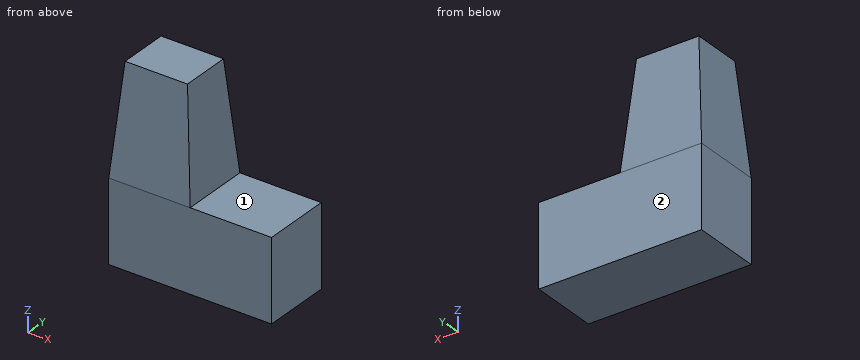
```python
from build123d import *

# Parameters (mm, degrees)
F0_W     = 60
F0_H     = 30
F1_DEPTH = 25.4
F2_W     = 30
F2_H     = 25.4
F3_DEPTH = 40
F3_TAPER = 5


with BuildPart() as f1:
    # F0 (on Front) → F1 (new body)
    with BuildSketch(Plane.XZ):
        with Locations((-10.6705549789, -15)):
            Rectangle(F0_W, F0_H)
    extrude(amount=F1_DEPTH)

    # F2 (on face) → F3 (join)
    with BuildSketch(Plane.XY):
        with Locations((-25.6705549789, -12.7)):
            Rectangle(F2_W, F2_H)
    extrude(amount=F3_DEPTH, taper=F3_TAPER)


solid = f1.part
```
Source: CAD feature listing. Evaluate the final solid. Frame: model axes, mm. Face numbers are marked on the shaded views. A direction names the side the tool comes from. Coordinates: 2 decimals unless noted, no trailing zeros. Loops run counter-clockwise (first coordinate to the right, second up) from the corner with the lowest first, then second, coordinate; pieces in that order, holes last. Notation, with made-up numbers: M -21.5,-32.75 L -10.5,-32.75 A24 ccw -10.5,-19.75 Z; hole C 68,-37 d11. An arc over 180 degrees is marked long. Put each result on its own line as item: value. Start each with the question number.
1) Cut plane D-D on x = 11. Return the cut outline in (y, z), then the cut area to 3 significant figures.
2) Reachability of the marked faces 1 and 2 from +Z, -Z, +X, -X, +Y, -Y: full face, straight path, thin tool, end or side. Return the list, or none.
3) Cut plane B-B on x = -26. Return the cut outline in (y, z).
4) Cut plane C-C on z = 14.5. Return the cut outline in (x, y), then the cut area to 3 significant figures.
5) Cut plane A-A on y = -16.75. Return the cut outline in (x, z).
6) Ray query, L1, parallel to Z at x = 8, y = -13.25; L2, parallel to X at y = -14.5, z = 12; L3, parallel to X at y = -13, z = 10.5. Return the intervals inside material, ascending. Write a range as from..to.
7) Contact query for flat-ended pins moving along their axis: pin 1 Ø4 at (y, z) = (-3, 11.5) entering from -X; pin 2 Ø3 at (x, y) = (-2.5, -16.5) entering from +Z; pin 3 Ø1 at (y, z) = (-18, 22.5) entering from -X. Output: stop coordinate, or through.
The answers:
1. outline: M -25.4,-30 L 0,-30 L 0,0 L -25.4,0 Z
1. area: 762 mm²
2. face 1: +Z, +X, +Y, -Y
2. face 2: +Z, -Z, +X, -X, +Y
3. outline: M -25.4,-30 L 0,-30 L 0,0 L -3.5,40 L -21.9,40 L -25.4,0 Z
4. outline: M -39.4,-24.13 L -11.94,-24.13 L -11.94,-1.27 L -39.4,-1.27 Z
4. area: 628 mm²
5. outline: M -40.67,-30 L 19.33,-30 L 19.33,0 L -10.67,0 L -14.17,40 L -37.17,40 L -40.67,0 Z
6. L1: z = -30..0
6. L2: x = -39.62..-11.72
6. L3: x = -39.75..-11.59
7. pin 1: stops at x = -39.84
7. pin 2: stops at z = 0
7. pin 3: stops at x = -38.75
